```python
from build123d import *

# Parameters (mm, degrees)
IZIM1_W                     = 10
IZIM1_H                     = 40
IZIM1_R                     = 2
Y_KSEKLIK_EKSTR_ZYON1_DEPTH = 2
IZIM2_R                     = 4
IZIM2_R_2                   = 1.937571625
Y_KSEKLIK_EKSTR_ZYON2_DEPTH = 4


with BuildPart() as part:
    # Çizim1 → Yükseklik-Ekstrüzyon1 (new body)
    with BuildSketch(Plane.XY):
        with Locations((5, 20)):
            Rectangle(IZIM1_W, IZIM1_H)
        with Locations((5, 20)):
            Circle(IZIM1_R, mode=Mode.SUBTRACT)
        with Locations((5, 33)):
            Circle(IZIM1_R, mode=Mode.SUBTRACT)
        with Locations(Location((5, 7, 0), (0, 0, 180))):
            Circle(IZIM1_R, mode=Mode.SUBTRACT)
    extrude(amount=Y_KSEKLIK_EKSTR_ZYON1_DEPTH)

    # Çizim2 → Yükseklik-Ekstrüzyon2 (add)
    with BuildSketch(Plane(origin=(0, 0, 0), x_dir=(-1, 0, 0), z_dir=(0, 0, -1))):
        with Locations((-5, 20)):
            Circle(IZIM2_R)
        with Locations((-5, 20)):
            Circle(IZIM2_R_2, mode=Mode.SUBTRACT)
    extrude(amount=Y_KSEKLIK_EKSTR_ZYON2_DEPTH)


solid = part.part
```
Geometry check sheet. Reference: the model listing, model coordinates, mm. A direction names the side the tool comes from. Give positions to 0.01 mm unless a question says otherwise; leave off trailing zeros. Order: outer loops, then holes, each group sorted by start corner. A loop starts at its lowest first (then second) coordinate and runs counter-clockwise, first axis right, second up. Notation, with made-up numbers: (40.5, 36.25) - (46.5, 36.25) arc R13 ccw to (46.5, 55.25) - close; hole circle Ø6 at (-1, 8). An arc over 180 degrees is marked (long way). Answer in a Markdown table with one row per item. Add a question column.
Q1. Cross-section at A-A, the plane x = 5. Enter the section's corners in (y, z).
Q2. Cross-section at B-B, the plane y = 7. Enter the section's corners in (x, z), then the cut area to 3 significant figures.
Q3. Material ranges on probe 1 along Y at (x, z) = (5, 0.8); probe 2 along Y at (x, z) = (5, -3.1); probe 3 along X at (y, z) = (7, 1.35), recorded low to high. Write a range as from..to.
Q4. Cross-section at D-D, the plane z = -0.45. Enter the section's corners in (x, y), then the cut area to 3 significant figures.
Q5. Tool access check on faces 4 (the flat face through (5, 40, 1)), 5 (the cylindrical face through (3.526, 21.352, 0.986)), 6 (the cylindrical face through (5.521, 23.966, -1.972)). Record the directions out of +Z, -Z, +X, -X, +Y, -Y that give a thin tool (end or side, any length) a straight path to the whole face; none if there is none.
Q6. Mould release check, pull along Y, two halves, no side actions. Record for faces 1 (the flat face through (5, 0, 1)), 2 (the cylindrical face through (5.42, 18.11, -1.97)), 3 (the flat face through (9.4, 20.3, 0)): pulls with the +Y half, pulls with the -Y half, needs draft (parallel to the pull), parting line crosses it, or undercut.
Q7. Gauge pin test, flat ends, axial feed: pin 1 (2 mm diameter, centred on y = 22, z = -3, fed in from +X); pin 2 (2 mm diameter, centred on x = 7.5, z = -1.5, fed in from -Y). Record the tip position at first contact, or that the pin passes through.
Q8. Cross-section at C-C, the plane z = 1.55. Enter the section's corners in (x, y), then the cut area to 3 significant figures.
Check values:
| question | item | result |
|---|---|---|
| 1 | outline | (0, 0) - (5, 0) - (5, 2) - (0, 2) - close; (9, 0) - (16, 0) - (16, -4) - (18.06, -4) - (18.06, 0) - (18, 0) - (18, 2) - (9, 2) - close; (21.94, -4) - (24, -4) - (24, 0) - (31, 0) - (31, 2) - (22, 2) - (22, 0) - (21.94, 0) - close; (35, 0) - (40, 0) - (40, 2) - (35, 2) - close |
| 2 | outline | (0, 0) - (3, 0) - (3, 2) - (0, 2) - close; (7, 0) - (10, 0) - (10, 2) - (7, 2) - close |
| 2 | area | 12.0 mm^2 |
| 3 | probe 1 | y = 0..5, 9..18, 22..31, 35..40 |
| 3 | probe 2 | y = 16..18.06, 21.94..24 |
| 3 | probe 3 | x = 0..3, 7..10 |
| 4 | outline | circle Ø8 at (5, 20); hole circle Ø3.88 at (5, 20) |
| 4 | area | 38.5 mm^2 |
| 5 | face 4 | +Z, -Z, +X, -X, +Y |
| 5 | face 5 | +Z |
| 5 | face 6 | -Z |
| 6 | face 1 | pulls with the -Y half |
| 6 | face 2 | undercut |
| 6 | face 3 | needs draft |
| 7 | pin 1 | stops at x = 8.87 |
| 7 | pin 2 | stops at y = 16.29 |
| 8 | outline | (0, 0) - (10, 0) - (10, 40) - (0, 40) - close; hole circle Ø4 at (5, 7); hole circle Ø4 at (5, 20); hole circle Ø4 at (5, 33) |
| 8 | area | 362 mm^2 |
